from build123d import *

# Parameters (mm, degrees)
RESSALTO_EXTRUS_O1_DEPTH = 5.9
RESSALTO_EXTRUS_O2_DEPTH = 2.9
ESBO_O3_R                = 1
CORTE_EXTRUS_O1_DEPTH    = 6.5


with BuildPart() as part:
    # Esboço1 → Ressalto-extrusão1 (new body)
    with BuildSketch(Plane.XY):
        with BuildLine():
            ThreePointArc((18.563238972, 0), (7.563238972, 11), (-3.436761028, 0))
            Line((-3.436761028, 0), (1.363238972, 0))
            ThreePointArc((1.363238972, 0), (7.563238972, 6.2), (13.763238972, 0))
            Line((13.763238972, 0), (18.563238972, 0))
        make_face()
    extrude(amount=RESSALTO_EXTRUS_O1_DEPTH)

    # Esboço2 → Ressalto-extrusão2 (add)
    with BuildSketch(Plane.XY.offset(5.9)):
        with BuildLine():
            ThreePointArc((-3.436761028, 0), (-3.390828585, 1.004193186), (-3.253414854, 2))
            Line((-3.253414854, 2), (-6.436761028, 2))
            Line((-6.436761028, 2), (-6.436761028, -2))
            Line((-6.436761028, -2), (-3.436761028, -2))
            Line((-3.436761028, -2), (-3.436761028, 0))
        make_face()
        with BuildLine():
            Line((-0.436761028, 2), (-3.253414854, 2))
            ThreePointArc((-3.253414854, 2), (-3.390828585, 1.004193186), (-3.436761028, 0))
            Line((-3.436761028, 0), (-0.436761028, 0))
            Line((-0.436761028, 0), (-0.436761028, 2))
        make_face()
        with BuildLine():
            ThreePointArc((18.379892799, 2), (18.517306529, 1.004193186), (18.563238972, 0))
            Line((18.563238972, 0), (18.563238972, -2))
            Line((18.563238972, -2), (21.563238972, -2))
            Line((21.563238972, -2), (21.563238972, 2))
            Line((21.563238972, 2), (18.379892799, 2))
        make_face()
        with BuildLine():
            Line((15.563238972, 0), (18.563238972, 0))
            ThreePointArc((18.563238972, 0), (18.517306529, 1.004193186), (18.379892799, 2))
            Line((18.379892799, 2), (15.563238972, 2))
            Line((15.563238972, 2), (15.563238972, 0))
        make_face()
    extrude(amount=-RESSALTO_EXTRUS_O2_DEPTH)

    # Esboço3 → Corte-extrusão1 (cut)
    with BuildSketch(Plane.XY.offset(5.9)):
        with Locations((20.063238972, 0)):
            Circle(ESBO_O3_R)
        with Locations((-4.936761028, 0)):
            Circle(ESBO_O3_R)
    extrude(amount=-CORTE_EXTRUS_O1_DEPTH, mode=Mode.SUBTRACT)


solid = part.part
Check sheet for the modelled part. Datum: model origin and axes. Units: mm. A direction names the side the tool comes from. Round coordinates to 2 decimals unless told otherwise and drop trailing zeros. Write each loop counter-clockwise with the first axis right and the second up, starting at its lowest first coordinate (ties: lowest second). Pieces come first, ordered by that corner, then holes. Notation, with made-up numbers: (35.25, 83.5) -> (58.25, 83.5) arc R19 ccw to (58.25, 113.5) -> close; hole circle Ø10 at (87, 68). An arc over 180 degrees is marked (long way). Answer as CSV lines item,"result". Start each with the question number.
1) Section check D-D on x = 5.5. Enter the section's corners in (y, z), and give its area (3 significant figures).
2) Go/stop test with flat-tipped pins: P1, Ø1.6, axis at x = 20, y = 0.5, coming from the -Z side; P2, Ø2.5, axis at x = -5.5, z = 4.5, coming from the +Y side; P3, Ø2.5, axis at x = 15.5, z = 2, coming from the -Y side; P4, Ø1.8, axis at x = -4.94, y = 0, coming from the -Z side. Record where each tip stops, or that it passes through.
3) Section check C-C on z = 1.1. Enter the section's corners in (x, y), and give its area (3 significant figures).
4) Release check for a two-part mould opening along X. For faces 5 (the cylindrical face through (7.805, 10.997, 2.909)), 6 (the flat face through (21.563, 0, 4)), 7 (the cylindrical face through (7.43, 6.2, 2.91)) record: pulls with the +X half, pulls with the -X half, needs draft (parallel to the pull), parting line crosses it, or undercut.
5) Section check B-B on y = 3. Enter the section's corners in (x, z).
6) Tool access check on faces 1 (the flat face through (-1, 0, 3)), 2 (the flat face through (20, -2, 4)), 3 (the flat face through (-5, 2, 4)), 4 (the flat face through (20, 2, 4)). Record the directions out of +Z, -Z, +X, -X, +Y, -Y that give a thin tool (end or side, any length) a straight path to the whole face; none if there is none.
7) Section check A-A on z = 5. Enter the section's corners in (x, y).
8) Material ranges on line 1 (Y direction, x = 19, z = 4.4); line 2 (X direction, y = 1, z = 2.85); line 3 (X direction, y = 1.5, z = 0.4), recorded low to high. Write a range as from..to.
Found:
1,outline,"(5.85, 0) -> (10.8, 0) -> (10.8, 5.9) -> (5.85, 5.9) -> close"
1,area,"29.3 mm^2"
2,P1,"stops at z = 3"
2,P2,"stops at y = 2"
2,P3,"stops at y = 0"
2,P4,"passes through"
3,outline,"(-3.44, 0) -> (1.36, 0) arc R6.2 cw to (13.76, 0) -> (18.56, 0) arc R11 ccw to start"
3,area,"130 mm^2"
4,face 5,"parting line crosses it"
4,face 6,"pulls with the +X half"
4,face 7,"undercut"
5,outline,"(-3.02, 0) -> (2.14, 0) -> (2.14, 5.9) -> (-3.02, 5.9) -> close; (12.99, 0) -> (18.15, 0) -> (18.15, 5.9) -> (12.99, 5.9) -> close"
6,face 1,"+Z, -Z, -Y"
6,face 2,"+Z, -Z, +X, -X, -Y"
6,face 3,"+Z, -Z, -X, +Y"
6,face 4,"+Z, -Z, +X, +Y"
7,outline,"(-6.44, -2) -> (-3.44, -2) -> (-3.44, 0) -> (1.36, 0) arc R6.2 cw to (13.76, 0) -> (18.56, 0) -> (18.56, -2) -> (21.56, -2) -> (21.56, 2) -> (18.38, 2) arc R11 ccw to (-3.25, 2) -> (-6.44, 2) -> close; hole circle Ø2 at (-4.94, 0); hole circle Ø2 at (20.06, 0)"
8,line 1,"y = -2..2"
8,line 2,"x = -3.39..1.44, 13.68..18.52"
8,line 3,"x = -3.33..1.55, 13.58..18.46"
